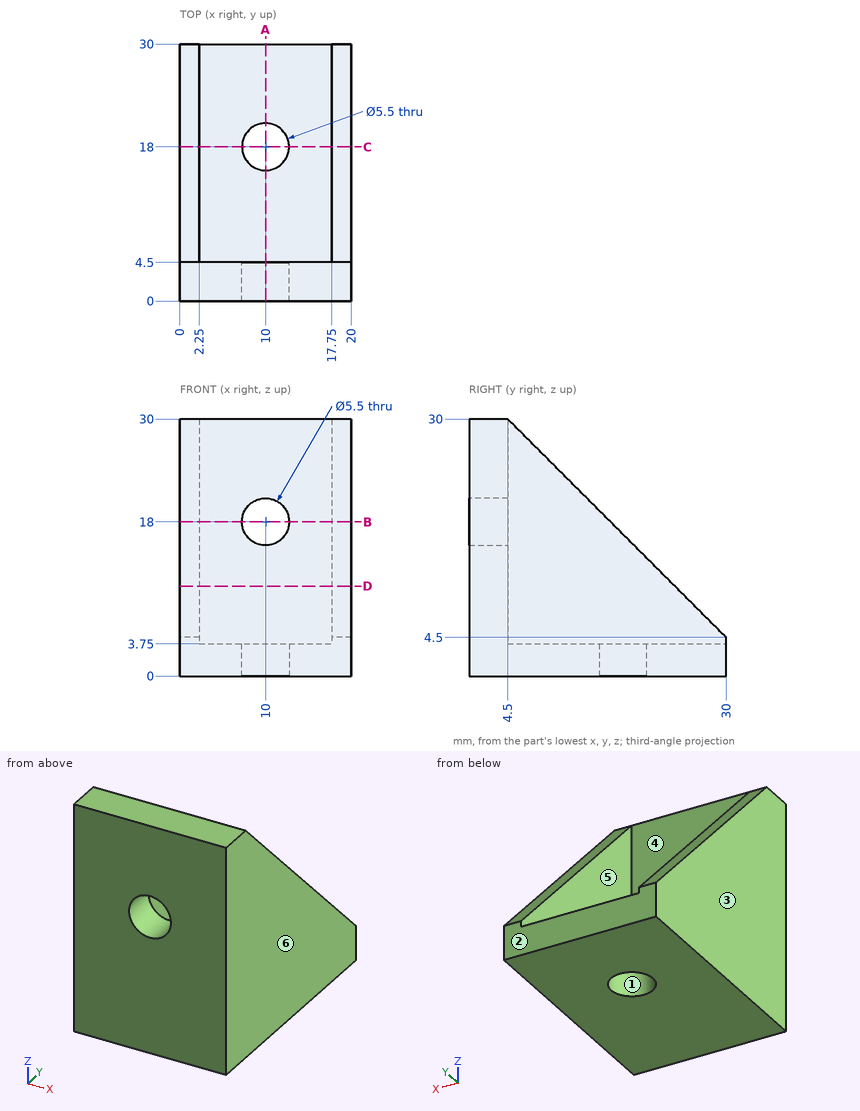
Job drawing, mm, ordinate dimensions from the low corner. One solid piece. A direction names the side the tool comes from. Round coordinates to 2 decimals unless told otherwise and drop trailing zeros. Loops run counter-clockwise (first coordinate to the right, second up) from the corner with the lowest first, then second, coordinate; pieces in that order, holes last.
Item 1: Drill centre lines: line 1 (Y direction, x = 10, z = 2.15); line 2 (X direction, y = 19.25, z = 6.5); line 3 (X direction, y = 3, z = 18). Where is each one in solid material? Low to high.
Item 2: Cut at B-B, the plane z = 18. Give the cut face in (x, y).
Item 3: Drop flat-ended pins along their axis: P1, Ø6.5, axis at x = 10, y = 18, coming from the +Z side; P2, Ø8, axis at x = 8, z = 12, coming from the +Y side; P3, Ø2, axis at x = 14.5, z = 4.5, coming from the -Y side; P4, Ø3.5, axis at x = 10, z = 18, coming from the -Y side. Give the stop position or say it passes through.
Item 4: Cut at A-A, the plane x = 10. Give the cut face in (y, z).
Item 5: Cut at C-C, the plane y = 18. Give the cut face in (x, z), then the cut area to 3 significant figures.
Item 6: Cut at D-D, the plane z = 10.5. Give the cut face in (x, y).
Item 7: 3-axis set-ups, long thin cutter, end or side, ignore diameter. For the marked faces 5 and 6: which of +Z, -Z, +X, -X, +Y, -Y reach the whole face in a straight line?
Item 8: Mould opens along X. For the marked faces 1, 2, 3 and 4 say: +X half, -X half, draft (parallel to the pull), parting line (faces both ways), or undercut.
A:
1. line 1: y = 0 to 15.25, 20.75 to 30
1. line 2: x = 0 to 2.25, 17.75 to 20
1. line 3: x = 0 to 7.25, 12.75 to 20
2. outline: (0, 0) - (7.25, 0) - (7.25, 4.5) - (2.25, 4.5) - (2.25, 16.5) - (0, 16.5) - close; (12.75, 0) - (20, 0) - (20, 16.5) - (17.75, 16.5) - (17.75, 4.5) - (12.75, 4.5) - close
3. P1: stops at z = 3.75
3. P2: stops at y = 4.5
3. P3: stops at y = 0
3. P4: passes through
4. outline: (0, 0) - (15.25, 0) - (15.25, 3.75) - (4.5, 3.75) - (4.5, 15.25) - (0, 15.25) - close; (0, 20.75) - (4.5, 20.75) - (4.5, 30) - (0, 30) - close; (20.75, 0) - (30, 0) - (30, 3.75) - (20.75, 3.75) - close
5. outline: (0, 0) - (7.25, 0) - (7.25, 3.75) - (2.25, 3.75) - (2.25, 16.5) - (0, 16.5) - close; (12.75, 0) - (20, 0) - (20, 16.5) - (17.75, 16.5) - (17.75, 3.75) - (12.75, 3.75) - close
5. area: 112 mm2
6. outline: (0, 0) - (20, 0) - (20, 24) - (17.75, 24) - (17.75, 4.5) - (2.25, 4.5) - (2.25, 24) - (0, 24) - close
7. face 5: +Z, +Y
7. face 6: +Z, -Z, +X, +Y, -Y
8. face 1: undercut
8. face 2: draft
8. face 3: -X half
8. face 4: undercut
